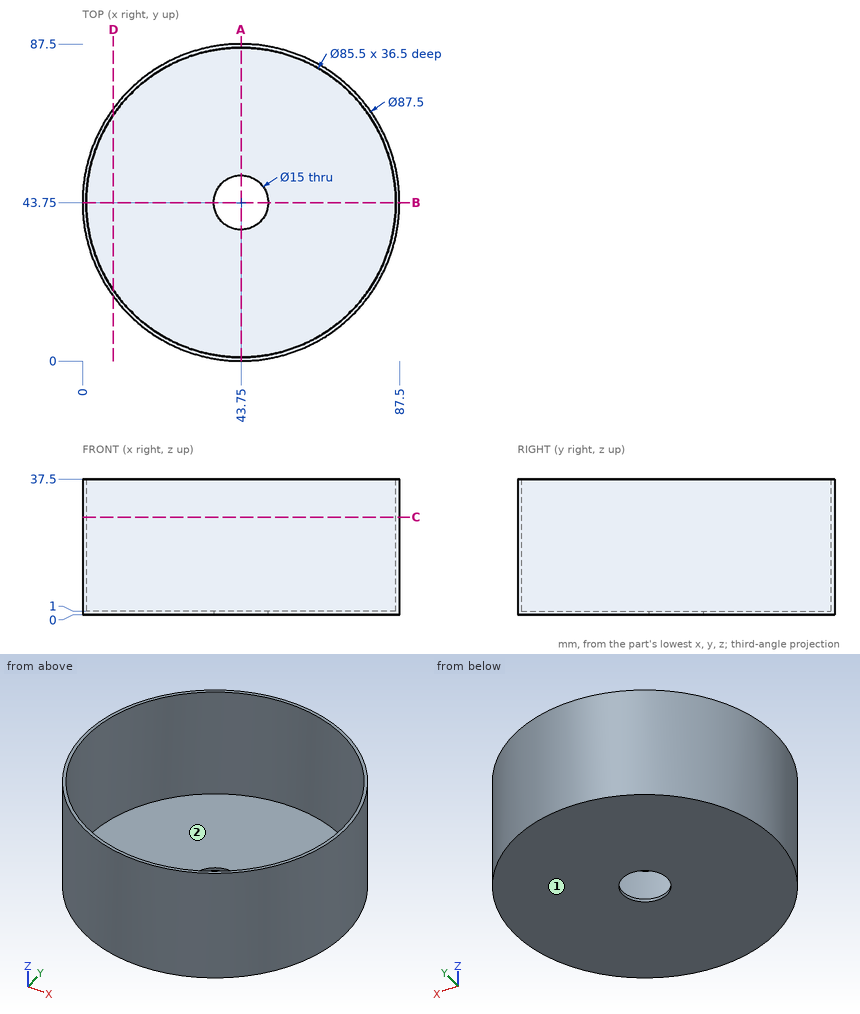
Here's the drawing with two shaded views (mm, measured from the low corner). I have some questions. A direction names the side the tool comes from. Coordinates: 2 decimals unless noted, no trailing zeros. Order: outer loops, then holes, each group sorted by start corner. A loop starts at its lowest first (then second) coordinate and runs counter-clockwise, first axis right, second up.
Q1. Suppose I cut it at C-C on z = 27. Please give me the cut outline in (x, y), and give its area (3 significant figures).
Q2. Suppose I cut it at D-D on x = 8.5. Please give me the cut outline in (y, z), and give its area (3 significant figures).
Q3. Which directions (+Z, -Z, +X, -X, +Y, -Y) give clear straight access to the entire face, cutting with the end or side of a thin tool? Please do the marked faces 1 and 2.
Q4. Please list where these lines run through material, in increasing order: L1, parallel to Y at x = 43.75, z = 28; L2, parallel to Z at x = 35, y = 82; L3, parallel to Y at x = 43.75, z = 0.25.
Q5. Suppose I cut it at A-A on x = 43.75. Please give me the cut outline in (y, z), and give its area (4 significant figures).
Q6. Will these pins go through, and if not, where does the flat tip stop? pin 1 (3 mm diameter, centred on y = 53.5, z = 6.5, fed in from -X); pin 2 (4 mm diameter, centred on y = 25, z = 10, fed in from +X); pin 3 (19.5 mm diameter, centred on x = 43.75, y = 43.75, fed in from +Z).
Answer:
1. outline: circle Ø87.5 at (43.75, 43.75); hole circle Ø85.5 at (43.75, 43.75)
1. area: 272 mm2
2. outline: (17.84, 0) - (69.66, 0) - (69.66, 37.5) - (67.94, 37.5) - (67.94, 1) - (19.56, 1) - (19.56, 37.5) - (17.84, 37.5) - close
2. area: 178 mm2
3. face 1: -Z, +X, -X, +Y, -Y
3. face 2: +Z
4. L1: y = 0 to 1, 86.5 to 87.5
4. L2: z = 0 to 1
4. L3: y = 0 to 36.25, 51.25 to 87.5
5. outline: (0, 0) - (36.25, 0) - (36.25, 1) - (1, 1) - (1, 37.5) - (0, 37.5) - close; (51.25, 0) - (87.5, 0) - (87.5, 37.5) - (86.5, 37.5) - (86.5, 1) - (51.25, 1) - close
5. area: 145.5 mm2
6. pin 1: stops at x = 0.78
6. pin 2: stops at x = 84.17
6. pin 3: stops at z = 1
